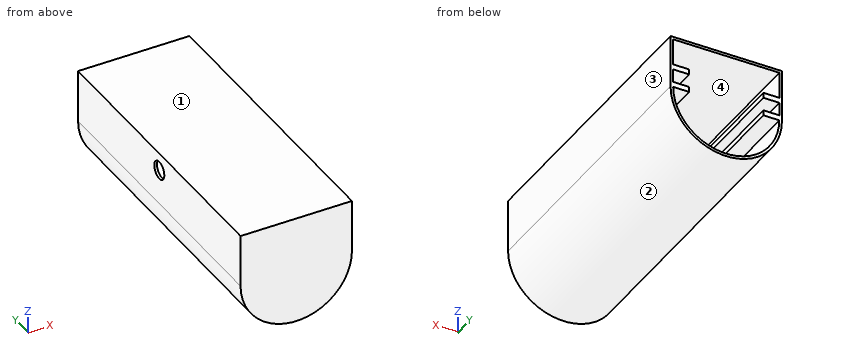
from build123d import *

# Parameters (mm, degrees)
BOSS_EXTRUDE1_DEPTH = 110
CUT_EXTRUDE1_DEPTH  = 109
SKETCH3_R           = 3.375
CUT_EXTRUDE2_DEPTH  = 5


with BuildPart() as part:
    # Sketch1 → Boss-Extrude1 (new body)
    with BuildSketch(Plane(origin=(0, 0, 0), x_dir=(1, 0, 0), z_dir=(0, 1, 0))):
        with BuildLine():
            Line((-40.883093525, -1.707733813), (1.116906475, -1.707733813))
            Line((1.116906475, -1.707733813), (1.116906475, 18.292266187))
            ThreePointArc((1.116906475, 18.292266187), (-19.883093525, 39.292266187), (-40.883093525, 18.292266187))
            Line((-40.883093525, 18.292266187), (-40.883093525, -1.707733813))
        make_face()
    extrude(amount=BOSS_EXTRUDE1_DEPTH)

    # Sketch2 → Cut-Extrude1 (cut)
    with BuildSketch(Plane(origin=(0, 110, 0), x_dir=(1, 0, 0), z_dir=(0, 1, 0))):
        with BuildLine():
            Line((-39.883093525, 16.292266187), (-39.883093525, 11.292266187))
            Line((-39.883093525, 11.292266187), (-33.883093525, 11.292266187))
            Line((-33.883093525, 11.292266187), (-33.883093525, 9.292266187))
            Line((-33.883093525, 9.292266187), (-39.883093525, 9.292266187))
            Line((-39.883093525, 9.292266187), (-39.883093525, -0.707733813))
            Line((-39.883093525, -0.707733813), (0.116906475, -0.707733813))
            Line((0.116906475, -0.707733813), (0.116906475, 9.292266187))
            Line((0.116906475, 9.292266187), (-5.883093525, 9.292266187))
            Line((-5.883093525, 9.292266187), (-5.883093525, 11.292266187))
            Line((-5.883093525, 11.292266187), (0.116906475, 11.292266187))
            Line((0.116906475, 11.292266187), (0.116906475, 16.292266187))
            Line((0.116906475, 16.292266187), (-5.883093525, 16.292266187))
            Line((-5.883093525, 16.292266187), (-5.883093525, 18.292266187))
            Line((-5.883093525, 18.292266187), (0.116906475, 18.292266187))
            ThreePointArc((0.116906475, 18.292266187), (-19.883093525, 38.292266187), (-39.883093525, 18.292266187))
            Line((-39.883093525, 18.292266187), (-33.883093525, 18.292266187))
            Line((-33.883093525, 18.292266187), (-33.883093525, 16.292266187))
            Line((-33.883093525, 16.292266187), (-39.883093525, 16.292266187))
        make_face()
    extrude(amount=-CUT_EXTRUDE1_DEPTH, mode=Mode.SUBTRACT)

    # Sketch3 → Cut-Extrude2 (cut)
    with BuildSketch(Plane.ZY.offset(40.883093525)):
        with Locations((-4.958932854, 55)):
            Circle(SKETCH3_R)
    extrude(amount=-CUT_EXTRUDE2_DEPTH, mode=Mode.SUBTRACT)


solid = part.part
Build history of the part. All positions in model axes, mm. Face numbers are marked on the shaded views. Round coordinates to 2 decimals unless told otherwise and drop trailing zeros. Order: outer loops, then holes, each group sorted by start corner. A loop starts at its lowest first (then second) coordinate and runs counter-clockwise, first axis right, second up. Notation, with made-up numbers: M 21,41 L 36,41 A17 ccw 36,69 Z; hole C 72,48.25 d7. An arc over 180 degrees is marked long. Use CSV: the item, a comma, the result in double quotes. Start each with the question number.
(1) Cut at A-A on y = 18. List the corners of the cut face in (x, z), then the cut area to 3 significant figures.
(2) Drill centre lines: probe 1 along X at (y, z) = (63.5, -15.5); probe 2 along Z at (x, y) = (-19, 36); probe 3 along Y at (x, z) = (-9, -33). Where is each one in solid material? Low to high.
(3) Flat gauge pins, fed straight in: P1, Ø4, axis at y = 14.5, z = -31.5, coming from the -X side; P2, Ø4, axis at x = -7, z = -23.5, coming from the +Y side; P3, Ø6, axis at x = -32, z = -8.5, coming from the -Y side; P4, Ø5, axis at x = -35.5, y = 28.5, coming from the -Z side. Where does each tip first touch, or does it go through?
(4) Cut at C-C on x = -17. List the corners of the cut face in (y, z), then the cut area to 3 significant figures.
(5) Cut at B-B on y = 55. List the corners of the cut face in (x, z).
(6) Cut at D-D on x = -23.5. List the corners of the cut face in (y, z).
(7) Mould opens along Z. For the marked faces 1, 2, 3 and 4 say: +Z half, -Z half, draft (parallel to the pull), parting line (faces both ways), or undercut.
Findings:
1,outline,"M -40.88,-18.29 A21 ccw 1.12,-18.29 L 1.12,1.71 L -40.88,1.71 Z; hole M -39.88,-18.29 A20 ccw 0.12,-18.29 L -5.88,-18.29 L -5.88,-16.29 L 0.12,-16.29 L 0.12,-11.29 L -5.88,-11.29 L -5.88,-9.29 L 0.12,-9.29 L 0.12,0.71 L -39.88,0.71 L -39.88,-9.29 L -33.88,-9.29 L -33.88,-11.29 L -39.88,-11.29 L -39.88,-16.29 L -33.88,-16.29 L -33.88,-18.29 Z"
1,area,"192 mm^2"
2,probe 1,"x = -40.88 to -39.88, 0.12 to 1.12"
2,probe 2,"z = -39.27 to -38.27, 0.71 to 1.71"
2,probe 3,"y = 0 to 1"
3,P1,"stops at x = -37.64"
3,P2,"stops at y = 1"
3,P3,"stops at y = 0"
3,P4,"stops at z = -34.69"
4,outline,"M 0,-39.09 L 110,-39.09 L 110,-38.08 L 1,-38.08 L 1,0.71 L 110,0.71 L 110,1.71 L 0,1.71 Z"
4,area,"260 mm^2"
5,outline,"M -40.88,-18.29 A21 ccw 1.12,-18.29 L 1.12,1.71 L -40.88,1.71 L -40.88,-1.58 L -39.88,-1.58 L -39.88,0.71 L 0.12,0.71 L 0.12,-9.29 L -5.88,-9.29 L -5.88,-11.29 L 0.12,-11.29 L 0.12,-16.29 L -5.88,-16.29 L -5.88,-18.29 L 0.12,-18.29 A20 cw -39.88,-18.29 L -33.88,-18.29 L -33.88,-16.29 L -39.88,-16.29 L -39.88,-11.29 L -33.88,-11.29 L -33.88,-9.29 L -39.88,-9.29 L -39.88,-8.33 L -40.88,-8.33 Z"
6,outline,"M 0,-38.98 L 110,-38.98 L 110,-37.96 L 1,-37.96 L 1,0.71 L 110,0.71 L 110,1.71 L 0,1.71 Z"
7,face 1,"+Z half"
7,face 2,"-Z half"
7,face 3,"draft"
7,face 4,"undercut"
